```python
from build123d import *

# Parameters (mm, degrees)
F2_DEPTH = 6.35
F3_DEPTH = 6.35


# Not quite as in the source:
# - a feature of the source that left no trace in its solid (it failed there, or was rolled back) is left out


with BuildPart() as f2:
    # F1 (on Top) → F2 (new body)
    with BuildSketch(Plane.XY):
        with BuildLine():
            ThreePointArc((14.2875, -8.248891971), (10.4591759131, 6.038608029), (0, 16.4977839421))
            ThreePointArc((0, 16.4977839421), (-10.4591759131, 6.038608029), (-14.2875, -8.248891971))
            ThreePointArc((-14.2875, -8.248891971), (0, -12.0772160579), (14.2875, -8.248891971))
        make_face()
    extrude(amount=F2_DEPTH)

    # F0 (on Top) → F3 (cut, through all)
    with BuildSketch(Plane.XY):
        with BuildLine():
            ThreePointArc((9.525, -5.499261314), (6.9727839421, 4.025738686), (0, 10.9985226281))
            ThreePointArc((0, 10.9985226281), (-6.9727839421, 4.025738686), (-9.525, -5.499261314))
            ThreePointArc((-9.525, -5.499261314), (0, -8.0514773719), (9.525, -5.499261314))
        make_face()
    extrude(amount=F3_DEPTH, mode=Mode.SUBTRACT)


solid = f2.part
```
For this review, take the finished solid that the model builds, in its own axes (mm). A direction names the side the tool comes from. Round coordinates to 2 decimals unless told otherwise and drop trailing zeros. Loops run counter-clockwise (first coordinate to the right, second up) from the corner with the lowest first, then second, coordinate; pieces in that order, holes last.
(1) We need section D-D (x = 11.75). Give the boundary of the cut face in (y, z).
Returned:
outline: (-9.55, 0) - (3.52, 0) - (3.52, 6.35) - (-9.55, 6.35) - close
(2) Tool access review of faces 1 (the cylindrical face through (-6.9, 4.15, 3.13)), 2 (the flat face through (-7, -7, 6.35)): name each direction out of +Z, -Z, +X, -X, +Y, -Y from which nothing blocks a thin tool from reaching the whole face with its end or side.
Returned:
face 1: +Z, -Z
face 2: +Z, +X, -X, +Y, -Y
(3) We need section C-C (x = -9). Give the boundary of the cut face in (y, z), plus the area to 3 significant figures.
Returned:
outline: (-10.62, 0) - (-5.79, 0) - (-5.79, 6.35) - (-10.62, 6.35) - close; (-1.06, 0) - (8.31, 0) - (8.31, 6.35) - (-1.06, 6.35) - close
area: 90.2 mm2
(4) Wall thickness on line 1 along X through (y, z) = (10.5, 4.25); line 2 along X through (y, z) = (9.25, 2); line 3 along Y through (x, z) = (-0.25, 3): over which ranges is each line inside the solid? List them lowest first.
Returned:
line 1: x = -7.28 to -0.82, 0.82 to 7.28
line 2: x = -8.3 to -2.53, 2.53 to 8.3
line 3: y = -12.08 to -8.05, 10.85 to 16.35
(5) We need section B-B (y = 6.5). Give the boundary of the cut face in (x, z).
Returned:
outline: (-10.19, 0) - (-5.27, 0) - (-5.27, 6.35) - (-10.19, 6.35) - close; (5.27, 0) - (10.19, 0) - (10.19, 6.35) - (5.27, 6.35) - close
(6) Mouldability with a two-part tool opening along X and no side actions: class faces 3 (the flat face through (-7, -7, 0)), 4 (the cylindrical face through (10.56, 5.86, 3.13)), 5 (the cylindrical face through (7.042, 3.905, 3.131)) as released by +X, released by -X, zero draft, split by the parting line, or undercut.
Returned:
face 3: zero draft
face 4: released by +X
face 5: undercut
(7) Clearance check with flat-ended pins moving along their axes: P1, Ø4, axis at x = 4, y = -5.5, coming from the -Z side; P2, Ø1, axis at x = 4.5, z = 1.5, coming from the -Y side; P3, Ø1, axis at y = -7, z = 4.5, coming from the -X side; P4, Ø3, axis at x = 9.5, z = 2, coming from the +Y side. State where each tip first meets the part, or that it passes through.
Returned:
P1: passes through
P2: stops at y = -11.8
P3: stops at x = -14.28
P4: stops at y = 9.63
